from build123d import *

# Parameters (mm, degrees)
PAD_DEPTH    = 10
SKETCH001_W  = 112.5
SKETCH001_H  = 11
PAD001_DEPTH = 10
POCKET_DEPTH = 10.5


with BuildPart() as part:
    # Sketch → Pad (new body)
    with BuildSketch(Plane.XY):
        Polygon((0, 0), (0, 2.51), (5, 2.51), (123.5, 2.51), (128.5, 2.51), (128.5, 0), align=None)
    extrude(amount=PAD_DEPTH)

    # Sketch001 → Pad001 (join)
    with BuildSketch(Plane.XY):
        with Locations((64.25, -4.5)):
            Rectangle(SKETCH001_W, SKETCH001_H)
    extrude(amount=PAD001_DEPTH)

    # Sketch002 → Pocket (cut, symmetric)
    with BuildSketch(Plane.XZ):
        with BuildLine():
            ThreePointArc((20, 16), (14, 10), (20, 4))
            Line((20, 4), (40, 4))
            ThreePointArc((40, 4), (46, 10), (40, 16))
            Line((40, 16), (20, 16))
        make_face()
    extrude(amount=POCKET_DEPTH, both=True, mode=Mode.SUBTRACT)


solid = part.part
For this review, take the finished solid that the model builds, in its own axes (mm). A direction names the side the tool comes from. Coordinates: 2 decimals unless noted, no trailing zeros. Order: outer loops, then holes, each group sorted by start corner. A loop starts at its lowest first (then second) coordinate and runs counter-clockwise, first axis right, second up. Notation, with made-up numbers: (-2.5, -15) -> (41.5, -15) arc R38 ccw to (41.5, 24) -> close; hole circle Ø11 at (87, 62). An arc over 180 degrees is marked (long way). Return JSON: item names as keys, results as strings.
1. We need section A-A on z = 2. Write out the cut boundary in (x, y).
Answer block:
{"outline": "(0, 0) -> (8, 0) -> (8, -10) -> (120.5, -10) -> (120.5, 0) -> (128.5, 0) -> (128.5, 2.51) -> (0, 2.51) -> close"}
2. We need section C-C on z = 8.5. Write out the cut boundary in (x, y), and give its area (3 significant figures).
Answer block:
{"outline": "(0, 0) -> (8, 0) -> (8, -10) -> (14.19, -10) -> (14.19, 2.51) -> (0, 2.51) -> close; (45.81, -10) -> (120.5, -10) -> (120.5, 0) -> (128.5, 0) -> (128.5, 2.51) -> (45.81, 2.51) -> close", "area": "1,050 mm²"}
3. We need section B-B on y = -8.75. Write out the cut boundary in (x, z).
Answer block:
{"outline": "(8, 0) -> (120.5, 0) -> (120.5, 10) -> (46, 10) arc R6 cw to (40, 4) -> (20, 4) arc R6 cw to (14, 10) -> (8, 10) -> close"}
4. Machinability: for faces 1 (the flat face through (4, 0, 5)), 2 (the cylindrical face through (44.196, -3.833, 5.711)), 3 (the flat face through (10, -2, 10)), 4 (the flat face through (120.5, -5, 5)), which of the approach directions +Z, -Z, +X, -X, +Y, -Y give a long, thin tool a straight path to every point of the face, cutting with its end or side? Answer none if there is none.
Answer block:
{"face 1": "+Z, -Z, -X, -Y", "face 2": "+Z, +Y, -Y", "face 3": "+Z, +X, -X, +Y, -Y", "face 4": "+Z, -Z, +X, -Y"}
5. For line 1 (X direction, y = -8.5, z = 3); line 2 (Z direction, x = 36, y = 0.5); line 3 (X direction, y = -0.5, z = 6), list the stretches that pass through material, from the lowest coordinate up. Write a range as from..to.
Answer block:
{"line 1": "8..120.5", "line 2": "0..4", "line 3": "8..15.53, 44.47..120.5"}
6. For pin 1 Ø4 at (x, z) = (5, 6.5) entering from -Y; pin 2 Ø3 at (y, z) = (-5.5, 7) entering from -X; pin 3 Ø2 at (y, z) = (-4.5, 4.5) entering from +X, all flat-tipped, find the tip position at first contact; note any pin that passes through.
Answer block:
{"pin 1": "y = 0", "pin 2": "x = 8", "pin 3": "x = 120.5"}
7. We need section D-D on x = 23.5. Write out the cut boundary in (y, z), and give its area (3 significant figures).
Answer block:
{"outline": "(-10, 0) -> (2.51, 0) -> (2.51, 4) -> (-10, 4) -> close", "area": "50.0 mm²"}
8. The part is to be moulded in two halves that separate along Y. For faces 5 (the flat face through (8, -5, 5)), 6 (the flat face through (65, 2.51, 5)), 7 (the flat face through (125, 0, 5)), say which applies: +Y half, -Y half, draft (parallel to the pull), parting line (faces both ways), or undercut.
Answer block:
{"face 5": "draft", "face 6": "+Y half", "face 7": "-Y half"}
